Job drawing, mm, ordinate dimensions from the low corner. One solid piece. A direction names the side the tool comes from. Give positions to 0.01 mm unless a question says otherwise; leave off trailing zeros. Write each loop counter-clockwise with the first axis right and the second up, starting at its lowest first coordinate (ties: lowest second). Pieces come first, ordered by that corner, then holes. Notation, with made-up numbers: (48.25, -18.75) -> (107.25, -18.75) arc R11 cw to (107.25, -3.75) -> close; hole circle Ø7 at (34, 60). An arc over 180 degrees is marked (long way). One line per question, with ' | ' between items. Start each with the question number.
(1) Tool access for the marked faces 4 and 5: list every direction of +Z, -Z, +X, -X, +Y, -Y with a clear straight run to the whole face (end or side of a thin tool).
(2) Drill centre lines: probe 1 along Y at (x, z) = (12.5, 1.3); probe 2 along Z at (x, y) = (22.5, 10); probe 3 along Y at (x, z) = (12.5, 11.75). Where is each one in solid material? Low to high. Write a range as from..to.
(3) Pin check, flat tips, straight feed: P1, Ø6, axis at y = 9.5, z = 7, coming from the +X side; P2, Ø8, axis at x = 11, y = 22, coming from the -Z side; P3, Ø4, axis at x = 20, y = 12.5, coming from the +Z side; P4, Ø8, axis at y = 7.5, z = 16.5, coming from the +X side. Stop position of each tip, or through.
(4) Pull direction Y, two halves, no side cores. Call the marked faces 1, 2 and 3: released by +Y, released by -Y, zero draft, split by the parting line, or undercut.
(5) Band-saw the part on C-C, the plane x = 12.5. Give the cut face in (y, z).
(6) Band-saw the part on A-A, the plane x = 20. Give the cut face in (y, z), and give its area (3 significant figures).
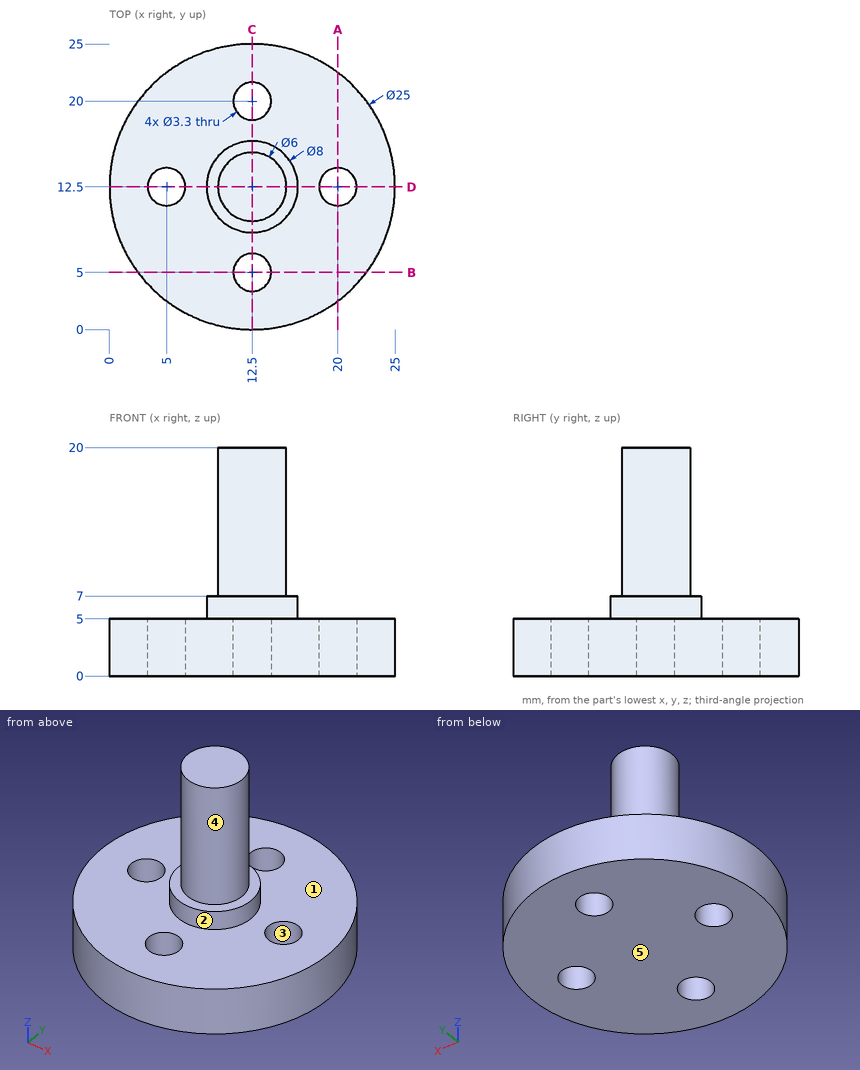
Results:
1) face 4: +Z | face 5: -Z, +X, -X, +Y, -Y
2) probe 1: y = 0..3.35, 6.65..18.35, 21.65..25 | probe 2: z = 0..5 | probe 3: y = 9.5..15.5
3) P1: stops at x = 24.98 | P2: stops at z = 0 | P3: stops at z = 5 | P4: stops at x = 15.33
4) face 1: zero draft | face 2: split by the parting line | face 3: undercut
5) outline: (0, 0) -> (3.35, 0) -> (3.35, 5) -> (0, 5) -> close; (6.65, 0) -> (18.35, 0) -> (18.35, 5) -> (16.5, 5) -> (16.5, 7) -> (15.5, 7) -> (15.5, 20) -> (9.5, 20) -> (9.5, 7) -> (8.5, 7) -> (8.5, 5) -> (6.65, 5) -> close; (21.65, 0) -> (25, 0) -> (25, 5) -> (21.65, 5) -> close
6) outline: (2.5, 0) -> (10.85, 0) -> (10.85, 5) -> (2.5, 5) -> close; (14.15, 0) -> (22.5, 0) -> (22.5, 5) -> (14.15, 5) -> close | area: 83.5 mm²
